```python
from build123d import *

# Parameters (mm, degrees)
EXTRUDE_1_DEPTH     = 20
SKETCH_3_OUTSIDE_W  = 154.97
SKETCH_3_OUTSIDE_H  = 154.97
SKETCH_3_OUTSIDE_R  = 22.5
CUT_EXTRUDE_2_DEPTH = 20
CUT_EXTRUDE_2_TAPER = 60
SKETCH_4_R          = 12.5
CUT_EXTRUDE_3_DEPTH = 21


with BuildPart() as part:
    # 草图1 → 凸台-拉伸1 (new body)
    with BuildSketch(Plane.XY):
        Polygon((22.5, -12.990381057), (22.5, 12.990381057), (0, 25.980762114), (-22.5, 12.990381057), (-22.5, -12.990381057), (0, -25.980762114), align=None)
    extrude(amount=EXTRUDE_1_DEPTH)

    # 草图2 → 旋转1 (revolve)
    with BuildSketch(Plane(origin=(0, 0, 0), x_dir=(0, 0, -1), z_dir=(1, 0, 0))):
        with BuildLine():
            Line((0, 0), (-12, 0))
            ThreePointArc((-12, 0), (-9.145772075, -17.058051419), (-0.894027207, -32.257802794))
            ThreePointArc((-0.894027207, -32.257802794), (-0.337232687, -32.42276506), (0, -31.95))
            Line((0, -31.95), (0, 0))
        make_face()
    revolve(axis=Axis((0, 0, 0), (0, 0, 1)))

    # 草图3 outside → 切除-拉伸2 (cut)
    with BuildSketch(Plane.XY.offset(20)):
        Rectangle(SKETCH_3_OUTSIDE_W, SKETCH_3_OUTSIDE_H)
        Circle(SKETCH_3_OUTSIDE_R, mode=Mode.SUBTRACT)
    extrude(amount=-CUT_EXTRUDE_2_DEPTH, taper=CUT_EXTRUDE_2_TAPER, mode=Mode.SUBTRACT)

    # 草图4 → 切除-拉伸3 (cut, through all)
    with BuildSketch(Plane.XY.offset(20)):
        Circle(SKETCH_4_R)
    extrude(amount=-CUT_EXTRUDE_3_DEPTH, mode=Mode.SUBTRACT)


solid = part.part
```
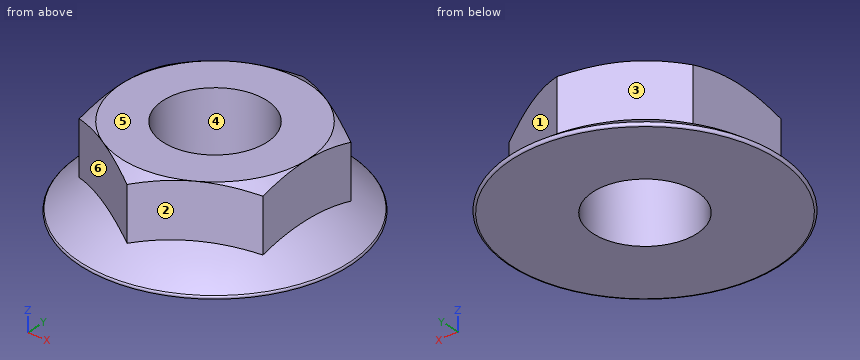
Geometry check sheet. Reference: the model listing, model coordinates, mm. Face numbers are marked on the shaded views. A direction names the side the tool comes from. Give positions to 0.01 mm unless a question says otherwise; leave off trailing zeros. Loops run counter-clockwise (first coordinate to the right, second up) from the corner with the lowest first, then second, coordinate; pieces in that order, holes last. Notation, with made-up numbers: M -5,57 L 10,57 A15 ccw 10,83 Z; hole C 10,-22.5 d1. An arc over 180 degrees is marked long. Write item = value, one per line.
(1) Release check for a two-part mould opening along X. For the marked faces 4, 5 and 6 record: released by +X, released by -X, zero draft, split by the parting line, or undercut.
Answer below:
face_4 = undercut
face_5 = zero draft
face_6 = released by -X
(2) Material ranges on line 1 (Y direction, x = 0, z = 16); line 2 (Y direction, x = -8.5, z = 7.5); line 3 (X direction, y = 9, z = 16), recorded low to high. Write a range as [from, to].
Answer below:
line_1 = [-25.98, -12.5], [12.5, 25.98]
line_2 = [-21.07, -9.17], [9.17, 21.07]
line_3 = [-22.5, -8.67], [8.67, 22.5]
(3) Gauge pin test, flat ends, axial feed: pin 1 Ø4.5 at (y, z) = (-0.5, 13.5) entering from -X; pin 2 Ø12 at (x, z) = (-15.5, 11) entering from +Y; pin 3 Ø20 at (x, y) = (0, 0) entering from -Z; pin 4 Ø10 at (x, z) = (-11.5, 8.5) entering from +Y. Record the tip position at first contact, or that the pin passes through.
Answer below:
pin_1 = -22.5
pin_2 = 21.72
pin_3 = through
pin_4 = 26.45
(4) Tool access check on the marked faces 1, 2 and 3. Record the directions out of +Z, -Z, +X, -X, +Y, -Y that give a thin tool (end or side, any length) a straight path to the whole face; none if there is none.
Answer below:
face_1 = +Z, +X, +Y
face_2 = +Z, +X, -Y
face_3 = +Z, -X, +Y
(5) Sectioned sample at A-A, the plane z = 14.5. Record the cut outline in (x, y), plus the area to 3 significant figures.
Answer below:
outline = M -22.5,-12.99 L 0,-25.98 L 22.5,-12.99 L 22.5,12.99 L 0,25.98 L -22.5,12.99 Z; hole C 0,0 d25
area = 1,260 mm2
(6) Sectioned sample at B-B, the plane z = 4. Record the cut outline in (x, y).
Answer below:
outline = C 0,0 d55.66; hole C 0,0 d25
